from build123d import *

# Parameters (mm, degrees)
PAD_DEPTH            = 170
PAD001_DEPTH         = 170
SKETCH003_W          = 7
SKETCH003_H          = 55
PAD002_DEPTH         = 29
POCKET_DEPTH         = 9
POCKET001_DEPTH      = 25
SKETCH005_R          = 1.4
POCKET002_DEPTH      = 7.001
SKETCH001_R          = 2
POCKET003_DEPTH      = 5
POCKET003_DEPTH_BACK = -100
POCKET004_DEPTH      = 40
PAD003_DEPTH         = 4
PAD004_DEPTH         = 61
POCKET005_DEPTH      = 5
POCKET005_DEPTH_BACK = -100
POCKET006_DEPTH      = 9
CHAMFER_SIZE         = 3
CHAMFER001_SIZE      = 1
FILLET_R             = 1
FILLET001_R          = 1


with BuildPart() as part:
    # Sketch → Pad (new body)
    with BuildSketch(Plane.XZ):
        with BuildLine():
            Line((0, 0), (2.5, 0))
            Line((2.5, 0), (2.5, -14))
            ThreePointArc((-8.875, -9.700654), (-6.298097, -20.080193), (2.5, -14))
            Line((-8.875, -9.700654), (-7, -11.354249))
            ThreePointArc((-7, -11.354249), (-5.414214, -17.741657), (0, -14))
            Line((0, 0), (0, -14))
        make_face()
    extrude(amount=PAD_DEPTH)

    # Sketch012 → Pad001 (join)
    with BuildSketch(Plane.XZ.offset(170)):
        Polygon((3.5, 0), (3.5, -13), (0.771706, -17.379086), (0.771706, 0), align=None)
    extrude(amount=-PAD001_DEPTH)

    # Sketch003 → Pad002 (join)
    with BuildSketch(Plane(origin=(2.5, 0, 0), x_dir=(0, 0, 1), z_dir=(1, 0, 0))):
        with Locations((-3.5, 142.5)):
            Rectangle(SKETCH003_W, SKETCH003_H)
    extrude(amount=PAD002_DEPTH)

    # Sketch008 → Pocket (cut)
    with BuildSketch(Plane(origin=(0, 0, 0), x_dir=(-1, 0, 0), z_dir=(0, 0, 1))):
        Polygon((-6, 171.390472), (-6, 155), (-43.587333, 117.412667), (-43.587333, 179.575119), align=None)
    extrude(amount=-POCKET_DEPTH, mode=Mode.SUBTRACT)

    # Sketch011 → Pocket001 (cut)
    with BuildSketch(Plane(origin=(34.5, 0, 0), x_dir=(0, 0, 1), z_dir=(1, 0, 0))):
        Polygon((-11.354396, 166.316992), (-3, 157.962596), (-3, 109.627052), (-19.434643, 110.990524), align=None)
    extrude(amount=-POCKET001_DEPTH, mode=Mode.SUBTRACT)

    # Sketch005 → Pocket002 (cut, through all)
    with BuildSketch(Plane(origin=(0, 0, -7), x_dir=(1, 0, 0), z_dir=(0, 0, -1))):
        with Locations((28, 120)):
            Circle(SKETCH005_R)
        with Locations((18, 120)):
            Circle(SKETCH005_R)
        with Locations((23, 128.660254)):
            Circle(SKETCH005_R)
    extrude(amount=-POCKET002_DEPTH, mode=Mode.SUBTRACT)

    # Sketch001 (on Face2 of Pad) → Pocket003 (cut, two sides)
    with BuildSketch(Plane(origin=(2.5, 0, 0), x_dir=(0, 0, 1), z_dir=(1, 0, 0))) as pocket003_sk:
        with Locations((-3.35, 12)):
            Circle(SKETCH001_R)
        with Locations((-3.35, 160)):
            Circle(SKETCH001_R)
        with BuildLine():
            ThreePointArc((-1.35, 6), (-3.35, 8), (-5.35, 6))
            Line((-5.35, 6), (-5.35, 4))
            ThreePointArc((-5.35, 4), (-3.35, 2), (-1.35, 4))
            Line((-1.35, 6), (-1.35, 4))
        make_face()
        with BuildLine():
            ThreePointArc((-1.35, 112.5), (-3.35, 114.5), (-5.35, 112.5))
            Line((-5.35, 112.5), (-5.35, 111.5))
            ThreePointArc((-5.35, 111.5), (-3.35, 109.5), (-1.35, 111.5))
            Line((-1.35, 112.5), (-1.35, 111.5))
        make_face()
        with BuildLine():
            ThreePointArc((-1.35, 62.5), (-3.35, 64.5), (-5.35, 62.5))
            Line((-5.35, 62.5), (-5.35, 61.5))
            ThreePointArc((-5.35, 61.5), (-3.35, 59.5), (-1.35, 61.5))
            Line((-1.35, 62.5), (-1.35, 61.5))
        make_face()
    extrude(amount=-POCKET003_DEPTH, mode=Mode.SUBTRACT)
    extrude(pocket003_sk.sketch, amount=-POCKET003_DEPTH_BACK, mode=Mode.SUBTRACT)

    # Sketch006 → Pocket004 (cut)
    with BuildSketch(Plane(origin=(0, 0, 0), x_dir=(1, 0, 0), z_dir=(0, 1, 0))):
        with BuildLine():
            ThreePointArc((-3.5, 5), (1.5, 10), (-3.5, 15))
            Line((-3.5, 15), (-3.5, 5))
        make_face()
    extrude(amount=-POCKET004_DEPTH, mode=Mode.SUBTRACT)

    # Sketch009 → Pad003 (join)
    with BuildSketch(Plane(origin=(0, 0, 0), x_dir=(1, 0, 0), z_dir=(0, 1, 0))):
        Polygon((-8.988888, 11.321152), (0, 11.321152), (0, 5.375637), (1.760757, 5.375637), (1.760757, 16.152864), (-3.184568, 19.176249), (-9.013494, 16.474098), align=None)
    extrude(amount=-PAD003_DEPTH)

    # Sketch010 → Pad004 (join)
    with BuildSketch(Plane.XZ.offset(170)):
        Polygon((1.607719, -11.392114), (-8.313037, -11.392114), (-9.514894, -14.319767), (-8.858657, -17.099121), (-6.117905, -19.22224), (-3.18414, -19.22224), (0.714678, -18.102777), (1.607719, -15.709445), align=None)
    extrude(amount=-PAD004_DEPTH)

    # Sketch004 → Pocket005 (cut, two sides)
    with BuildSketch(Plane(origin=(2.5, 0, 0), x_dir=(0, 0, 1), z_dir=(1, 0, 0))) as pocket005_sk:
        Polygon((-9.5, 109.884079), (-7.5, 107.884079), (-7.5, 100.23037), (1.897298, 90.833072), (4.794627, 81.589452), (-11.5, 97.884079), (-11.5, 107.884079), align=None)
    extrude(amount=-POCKET005_DEPTH, mode=Mode.SUBTRACT)
    extrude(pocket005_sk.sketch, amount=-POCKET005_DEPTH_BACK, mode=Mode.SUBTRACT)

    # Sketch013 (on Face63 of Pocket005) → Pocket006 (cut)
    with BuildSketch(Plane(origin=(0, 0, 0), x_dir=(-1, 0, 0), z_dir=(0, 0, 1))):
        Polygon((-3.5, 112.04879), (-3.5, 116.943748), (-13.285114, 112.394318), align=None)
    extrude(amount=-POCKET006_DEPTH, mode=Mode.SUBTRACT)

    # Chamfer
    chamfer_edges = [part.edges().sort_by_distance(p)[0] for p in [
        (31.5, -115, -1.5),
    ]]
    chamfer(chamfer_edges, length=CHAMFER_SIZE)

    # Chamfer001
    chamfer001_edges = [part.edges().sort_by_distance(p)[0] for p in [
        (6, -155, -3.5),
    ]]
    chamfer(chamfer001_edges, length=CHAMFER001_SIZE)

    # Fillet
    fillet_edges = [part.edges().sort_by_distance(p)[0] for p in [
        (9.5, -133.25, -3),
    ]]
    fillet(fillet_edges, radius=FILLET_R)

    # Fillet001
    fillet001_edges = [part.edges().sort_by_distance(p)[0] for p in [
        (9.5, -133.25, -7),
    ]]
    fillet(fillet001_edges, radius=FILLET001_R)


solid = part.part
For this review, take the finished solid that the model builds, in its own axes (mm). A direction names the side the tool comes from. Round coordinates to 2 decimals unless told otherwise and drop trailing zeros. Order: outer loops, then holes, each group sorted by start corner. A loop starts at its lowest first (then second) coordinate and runs counter-clockwise, first axis right, second up. Notation, with made-up numbers: M -15.5,26.25 L 0.5,26.25 A30 cw 0.5,49.25 Z; hole C 12.25,36.5 d2. An arc over 180 degrees is marked long. Use a Markdown table: item, result. Add a question column.
Item 1: Add section A-A, the plane y = -12. Give the boundary of the cut face in (x, z) (3 decimals).
Item 2: Tool access review of faces 4 (the cylindrical face through (1.5, -21.7, -9.9)), 5 (the cylindrical face through (1.8, -64.5, -3.3)), 6 (the flat face through (2, -103, -11.5)), 7 (the flat face through (18, -115, -2)): name each direction out of +Z, -Z, +X, -X, +Y, -Y from which nothing blocks a thin tool from reaching the whole face with its end or side.
Item 3: Insertion check: pin 1 (17 mm diameter, centred on x = 24.5, y = -131.5, fed in from -Z); pin 2 (7 mm diameter, centred on y = -49, z = -6.5, fed in from -X); pin 3 (3 mm diameter, centred on x = 2.5, y = -104.5, fed in from -Z); pin 4 (3.5 mm diameter, centred on y = -12, z = -3.35, fed in from -X). Each pin has a flat end and moves straight along its axis. Give the tip position at first contact, or say it passes through.
Item 4: Add section B-B, the plane x = -4. Give the boundary of the cut face in (y, z), then the cut area to 3 significant figures.
Item 5: To check wall thickness, follow line 1 along Y through (x, z) = (-2, -11.5); line 2 along Z through (x, y) = (4.5, -160); line 3 along X through (y, z) = (-59, -3.25). State the ranges of each line that lie inside material, in increasing order.
Item 6: Mouldability with a two-part tool opening along X and no side actions: class faces 1 (the flat face through (-2, -170, -12)), 2 (the flat face through (-4, -2, -11.321)), 3 (the cylindrical face through (-6.76, -83.81, -19.885)) as released by +X, released by -X, zero draft, split by the parting line, or undercut.
Geometry results:
| question | item | result |
|---|---|---|
| 1 | outline | M -8.875,-9.701 A6.5 ccw long 2.467,-14.659 L 3.5,-13 L 3.5,-5.35 L 0,-5.35 L 0,-6.429 A5 cw 0,-13.571 L 0,-14 A4 cw long -7,-11.354 Z; M 0,-1.35 L 3.5,-1.35 L 3.5,0 L 0,0 Z |
| 2 | face 4 | none |
| 2 | face 5 | +X, -X |
| 2 | face 6 | +X |
| 2 | face 7 | +Z, -Z, +X, +Y |
| 3 | pin 1 | stops at z = -3 |
| 3 | pin 2 | stops at x = -9.12 |
| 3 | pin 3 | stops at z = -18.15 |
| 3 | pin 4 | passes through |
| 4 | outline | M -170,-20.5 L 0,-20.5 L 0,-11.32 L -4,-11.32 L -4,-18 L -109,-18 L -109,-11.39 L -170,-11.39 Z |
| 4 | area | 855 mm² |
| 5 | line 1 | y = -170 to -109, -4 to 0 |
| 5 | line 2 | z = -7 to -5.35, -1.35 to 0 |
| 5 | line 3 | x = 0 to 3.5 |
| 6 | face 1 | zero draft |
| 6 | face 2 | undercut |
| 6 | face 3 | split by the parting line |
